Input: part model. Units: mm. Frame: model coordinates. Round coordinates to 2 decimals unless told otherwise and drop trailing zeros. Write each loop counter-clockwise with the first axis right and the second up, starting at its lowest first coordinate (ties: lowest second). Pieces come first, ordered by that corner, then holes. Notation, with made-up numbers: (12, 19) -> (20, 19) arc R26 cw to (20, 38) -> close; hole circle Ø11 at (30.25, 40). An arc over 180 degrees is marked (long way). Write item = value, one per line. Start each with the question number.
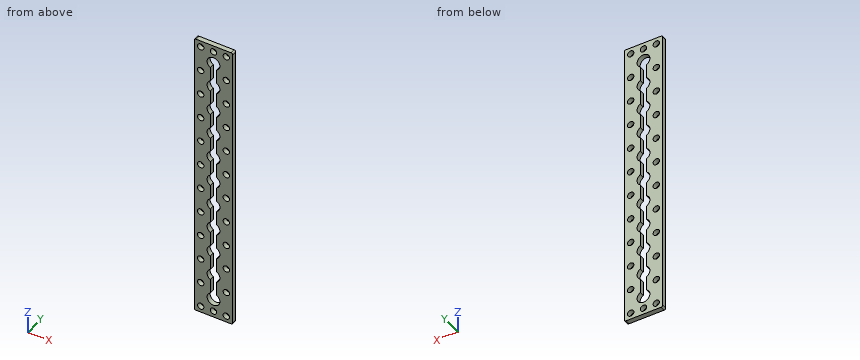
```python
from build123d import *

# Parameters (mm, degrees)
SKETCH1_W                = 24
SKETCH1_H                = 184
BOSS_EXTRUDE1_DEPTH      = 3
F_4_0_4_DIAMETER_HOLE1_D = 4
F_8_0_8_DIAMETER_HOLE1_D = 8
LPATTERN1_COUNT          = 11
LPATTERN1_PITCH          = 16
SKETCH9_W                = 4
SKETCH9_H                = 160
CUT_EXTRUDE1_DEPTH       = 3
FILLET1_R                = 1


with BuildPart() as part:
    # Sketch1 → Boss-Extrude1 (new body)
    with BuildSketch(Plane(origin=(0, 0, 0), x_dir=(1, 0, 0), z_dir=(0, 1, 0))):
        Rectangle(SKETCH1_W, SKETCH1_H)
    extrude(amount=BOSS_EXTRUDE1_DEPTH)

    # Ø4.0 (4) Diameter Hole1 (through all)
    with Locations(Plane(origin=(0, 3, 0), x_dir=(1, 0, 0), z_dir=(0, 1, 0))):
        with Locations((-8, 88), (0, 88), (8, 88), (-8, 72), (-8, 56), (8, 56), (8, 72), (-8, 40), (8, 40), (-8, 24), (-8, 8), (8, 8), (8, 24)):
            f_4_0_4_diameter_hole1 = Hole(F_4_0_4_DIAMETER_HOLE1_D / 2)

    # Mirror1: Ø4.0 (4) Diameter Hole1 across plane
    add(f_4_0_4_diameter_hole1.mirror(Plane.XY), mode=Mode.SUBTRACT)

    # Ø8.0 (8) Diameter Hole1 (through all)
    with Locations(Plane(origin=(0, 3, 0), x_dir=(1, 0, 0), z_dir=(0, 1, 0))):
        with Locations((0, 80)):
            f_8_0_8_diameter_hole1 = Hole(F_8_0_8_DIAMETER_HOLE1_D / 2)

    # LPattern1: Ø8.0 (8) Diameter Hole1 ×11
    with Locations(*[(0, 0, i * LPATTERN1_PITCH) for i in range(1, LPATTERN1_COUNT)]):
        add(f_8_0_8_diameter_hole1, mode=Mode.SUBTRACT)

    # Sketch9 → Cut-Extrude1 (cut)
    with BuildSketch(Plane(origin=(0, 3, 0), x_dir=(1, 0, 0), z_dir=(0, 1, 0))):
        Rectangle(SKETCH9_W, SKETCH9_H)
    extrude(amount=-CUT_EXTRUDE1_DEPTH, mode=Mode.SUBTRACT)

    # Fillet1
    fillet1_edges = [part.edges().sort_by_distance(p)[0] for p in [
        (-12, 1.5, -92),
        (12, 1.5, -92),
        (12, 1.5, 92),
        (-12, 1.5, 92),
    ]]
    fillet(fillet1_edges, radius=FILLET1_R)


solid = part.part
```
1. Section C-C (y = 1.95). State how many separate pieces and enclosed holes the cut face has, then the cut area to 3 significant figures.
2. Section A-A (z = -56). Output: boundary loops of the cut face in (x, y), then the cut area to 3 significant figures.
3. Section B-B (z = -80). Output: boundary loops of the cut face in (x, y), then the cut area to 3 significant figures.
4. Line query: line 1 along X through (y, z) = (1.9, -88); line 2 along X through (y, z) = (1.45, 80); line 3 along X through (y, z) = (1.8, -59). Output: solid intervals per line, ascending.
Check sheet entries:
q1.separate_pieces = 1
q1.enclosed_holes = 27
q1.area = 3,200 mm2
q2.outline = (-12, 0) -> (-10, 0) -> (-10, 3) -> (-12, 3) -> close; (-6, 0) -> (-2, 0) -> (-2, 3) -> (-6, 3) -> close; (2, 0) -> (6, 0) -> (6, 3) -> (2, 3) -> close; (10, 0) -> (12, 0) -> (12, 3) -> (10, 3) -> close
q2.area = 36.0 mm2
q3.outline = (-12, 0) -> (-4, 0) -> (-4, 3) -> (-12, 3) -> close; (4, 0) -> (12, 0) -> (12, 3) -> (4, 3) -> close
q3.area = 48.0 mm2
q4.line_1 = -12 to -10, -6 to -2, 2 to 6, 10 to 12
q4.line_2 = -12 to -4, 4 to 12
q4.line_3 = -12 to -2, 2 to 12
